Source: three-view drawing plus pictorial views. Frame: mm from the lowest corner of the part. A direction names the side the tool comes from. Give positions to 0.01 mm unless a question says otherwise; leave off trailing zeros. Loops run counter-clockwise (first coordinate to the right, second up) from the corner with the lowest first, then second, coordinate; pieces in that order, holes last.
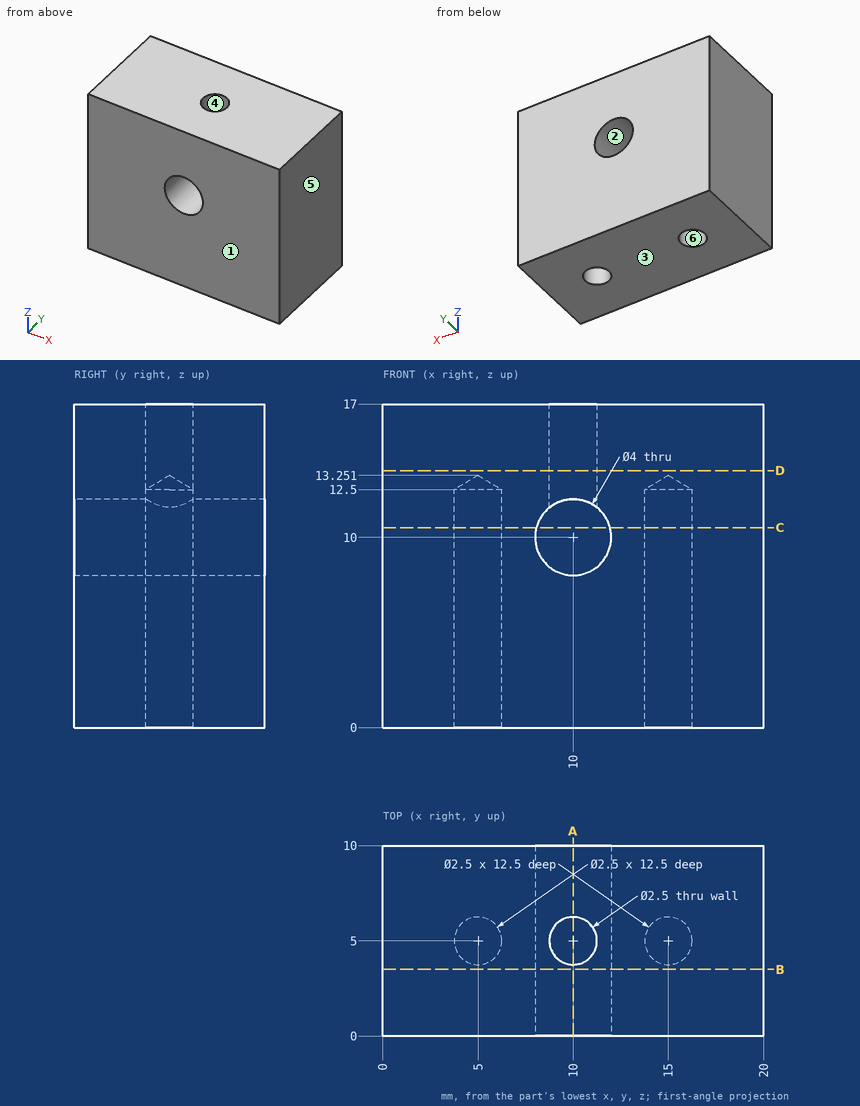
(1) Cut plane A-A (x = 10). Return the cut outline in (y, z).
Values follow:
outline: (0, 0) - (10, 0) - (10, 8) - (0, 8) - close; (0, 12) - (3.75, 12) - (3.75, 17) - (0, 17) - close; (6.25, 12) - (10, 12) - (10, 17) - (6.25, 17) - close
(2) Cut plane B-B (y = 3.5). Return the cut outline in (x, z), and give its area (3 significant figures).
Values follow:
outline: (0, 0) - (20, 0) - (20, 17) - (0, 17) - close; hole circle Ø4 at (10, 10)
area: 327 mm2
(3) Mould query, pull axis Z, two halves, no side actions, for the marked faces 1, 2 and 3. Classes: +Z half, -Z half, draft (parallel to the pull), parting line (faces both ways), or undercut.
Values follow:
face 1: draft
face 2: undercut
face 3: -Z half
(4) Cut plane C-C (z = 10.5). Return the cut outline in (x, y), and give its area (3 significant figures).
Values follow:
outline: (0, 0) - (8.06, 0) - (8.06, 10) - (0, 10) - close; (11.94, 0) - (20, 0) - (20, 10) - (11.94, 10) - close; hole circle Ø2.5 at (5, 5); hole circle Ø2.5 at (15, 5)
area: 151 mm2
(5) Ray query, probe 1 along Z at (x, y) = (10, 9.5); probe 2 along Y at (x, z) = (5, 7.5); probe 3 along X at (y, z) = (4.5, 9). Return the intervals inside material, ascending.
Values follow:
probe 1: z = 0 to 8, 12 to 17
probe 2: y = 0 to 3.75, 6.25 to 10
probe 3: x = 0 to 3.85, 6.15 to 8.27, 11.73 to 13.85, 16.15 to 20
(6) Pin query (flat end, axial travel): pin 1 Ø3.5 at (x, z) = (10, 10) entering from +Y. Return the tip coordinate at first contact, or that it passes through.
Values follow:
pin 1: passes through
(7) Cut plane D-D (z = 13.5). Return the cut outline in (x, y).
Values follow:
outline: (0, 0) - (20, 0) - (20, 10) - (0, 10) - close; hole circle Ø2.5 at (10, 5)
(8) Reachability of the marked faces 4, 5 and 6 from +Z, -Z, +X, -X, +Y, -Y: full face, straight path, thin tool, end or side. Return the list, or none.
Values follow:
face 4: +Z
face 5: +Z, -Z, +X, +Y, -Y
face 6: -Z
